from build123d import *

# Parameters (mm, degrees)
SKETCH_1_R      = 1.5
EXTRUDE_1_DEPTH = 3
FILLET_1_R      = 2


with BuildPart() as part:
    # 草图1 → 凸台-拉伸1 (new body)
    with BuildSketch(Plane(origin=(0, 0, 0), x_dir=(1, 0, 0), z_dir=(0, 1, 0))):
        with BuildLine():
            Line((-52.5, 20), (-52.5, -20))
            Line((-52.5, -20), (-37.5, -20))
            ThreePointArc((-37.5, -20), (-35.303300859, -14.696699141), (-30, -12.5))
            Line((-30, -12.5), (-12.708053938, -12.5))
            Line((-12.708053938, -12.5), (-10.673252989, -4.338859148))
            ThreePointArc((-10.673252989, -4.338859148), (0, 4), (10.673252989, -4.338859148))
            Line((10.673252989, -4.338859148), (12.708053938, -12.5))
            Line((12.708053938, -12.5), (30, -12.5))
            ThreePointArc((30, -12.5), (35.303300859, -14.696699141), (37.5, -20))
            Line((37.5, -20), (52.5, -20))
            Line((52.5, -20), (52.5, 20))
            Line((52.5, 20), (37.5, 20))
            ThreePointArc((37.5, 20), (35.303300859, 14.696699141), (30, 12.5))
            Line((30, 12.5), (-30, 12.5))
            ThreePointArc((-30, 12.5), (-35.303300859, 14.696699141), (-37.5, 20))
            Line((-37.5, 20), (-52.5, 20))
        make_face()
        with Locations(Location((-44.901280605, 15, 0), (0, 0, 270))):
            Circle(SKETCH_1_R, mode=Mode.SUBTRACT)
        with Locations(Location((-44.901280605, -15, 0), (0, 0, 270))):
            Circle(SKETCH_1_R, mode=Mode.SUBTRACT)
        with Locations(Location((44.901280605, -15, 0), (0, 0, 270))):
            Circle(SKETCH_1_R, mode=Mode.SUBTRACT)
        with Locations(Location((44.901280605, 15, 0), (0, 0, 270))):
            Circle(SKETCH_1_R, mode=Mode.SUBTRACT)
        with Locations(Location((15, 9, 0), (0, 0, 270))):
            Circle(SKETCH_1_R, mode=Mode.SUBTRACT)
        with Locations(Location((15, -9, 0), (0, 0, 270))):
            Circle(SKETCH_1_R, mode=Mode.SUBTRACT)
        with Locations(Location((-15, 9, 0), (0, 0, 270))):
            Circle(SKETCH_1_R, mode=Mode.SUBTRACT)
        with Locations(Location((-15, -9, 0), (0, 0, 270))):
            Circle(SKETCH_1_R, mode=Mode.SUBTRACT)
    extrude(amount=EXTRUDE_1_DEPTH)

    # 圆角1
    fillet_1_edges = [part.edges().sort_by_distance(p)[0] for p in [
        (12.708053938, 1.5, 12.5),
        (-12.708053938, 1.5, 12.5),
    ]]
    fillet(fillet_1_edges, radius=FILLET_1_R)


solid = part.part
Could you check a few things on this model? Use its own coordinates, in mm. A direction names the side the tool comes from. Coordinates: 2 decimals unless noted, no trailing zeros. Write each loop counter-clockwise with the first axis right and the second up, starting at its lowest first coordinate (ties: lowest second). Pieces come first, ordered by that corner, then holes. Notation, with made-up numbers: M 24,35.25 L 47,35.25 A25 ccw 47,74.25 Z; hole C 45.25,-18.5 d6. An arc over 180 degrees is marked long. One line per question, with ' | ' between items.
1) If we mould it in two halves opening along X, with no side actions, what happens to faces 1 (the face through (-45, 1, 20)), 2 (the face through (-52.5, 1, 0)), 3 (the face through (-43.414, 1.479, -15.195)), 4 (the face through (-35.245, 1.479, -14.639))? For each: released by +X, released by -X, zero draft, split by the parting line, or undercut.
Checks:
face 1: zero draft | face 2: released by -X | face 3: undercut | face 4: undercut
2) Imagine slicing it at C-C, the plane z = -0.5. Write out the boundary of the cut face in (x, y).
Checks:
outline: M -52.5,0 L -8.05,0 L -8.05,3 L -52.5,3 Z; M 8.05,0 L 52.5,0 L 52.5,3 L 8.05,3 Z
3) For faces 5 (the face through (35.361, 1.479, -14.755)), 6 (the face through (43.44, 1.48, -15.33)), 7 (the face through (22, 1, 12.5)), which set-ups out of +Z, -Z, +X, -X, +Y, -Y let a thin tool reach every point of the face, with its end or its side?
Checks:
face 5: -Z, +Y, -Y | face 6: +Y, -Y | face 7: +Z, +Y, -Y
4) Imagine slicing it at B-B, the plane y = 1.05. Give the number of separate pieces and of enclosed holes in the cut face, and give its area (3 significant figures).
Checks:
separate pieces: 1 | enclosed holes: 8 | area: 2,740 mm²
5) Imagine slicing it at A-A, the plane z = 15. Write out the boundary of the cut face in (x, y), and give its area (3 significant figures).
Checks:
outline: M -52.5,0 L -46.4,0 L -46.4,3 L -52.5,3 Z; M -43.4,0 L -35.59,0 L -35.59,3 L -43.4,3 Z; M 35.59,0 L 43.4,0 L 43.4,3 L 35.59,3 Z; M 46.4,0 L 52.5,0 L 52.5,3 L 46.4,3 Z | area: 83.5 mm²
6) Imagine slicing it at D-D, the plane x = 36. Write out the boundary of the cut face in (y, z), and give its area (3 significant figures).
Checks:
outline: M 0,-15.5 L 3,-15.5 L 3,15.5 L 0,15.5 Z | area: 93.0 mm²
7) I need wall thicknesses on probe 1 along X at (y, z) = (1.6, -9); probe 2 along X at (y, z) = (2.4, 9); probe 3 along X at (y, z) = (1.8, 15). Which ranges of each line are inside material? Lowest first, please. Write a range as [from, to].
Checks:
probe 1: [-52.5, -16.5], [-13.5, 13.5], [16.5, 52.5] | probe 2: [-52.5, -16.5], [-13.5, -11.84], [11.84, 13.5], [16.5, 52.5] | probe 3: [-52.5, -46.4], [-43.4, -35.59], [35.59, 43.4], [46.4, 52.5]
8) For pin 1 Ø0.9 at (x, y) = (-21.5, 1) entering from +Z, with a flat end and sliding along its axis, tell me the tip position at first contact or that it passes through.
Checks:
pin 1: z = 12.5
